Build history of the part. All positions in model axes, mm. Give positions to 0.01 mm unless a question says otherwise; leave off trailing zeros. Loops run counter-clockwise (first coordinate to the right, second up) from the corner with the lowest first, then second, coordinate; pieces in that order, holes last. Notation, with made-up numbers: M 87,17.5 L 118,17.5 A10 ccw 118,22.5 Z; hole C 66,-40 d9. An arc over 180 degrees is marked long. Put each result on its own line as item: value.
```python
from build123d import *

# Parameters (mm, degrees)
SKETCH1_R           = 4
SKETCH1_R_2         = 12
BOSS_EXTRUDE1_DEPTH = 2.5
FILLET1_R           = 4


with BuildPart() as part:
    # Sketch1 → Boss-Extrude1 (new, symmetric)
    with BuildSketch(Plane(origin=(0, 0, 0), x_dir=(1, 0, 0), z_dir=(0, 1, 0))):
        with BuildLine():
            Line((39.081081081, 10.801347209), (3.405405405, 17.674931797))
            ThreePointArc((3.405405405, 17.674931797), (0, 18), (-3.405405405, 17.674931797))
            Line((-3.405405405, 17.674931797), (-39.081081081, 10.801347209))
            ThreePointArc((-39.081081081, 10.801347209), (-48, 0), (-39.081081081, -10.801347209))
            Line((-39.081081081, -10.801347209), (-3.405405405, -17.674931797))
            ThreePointArc((-3.405405405, -17.674931797), (0, -18), (3.405405405, -17.674931797))
            Line((3.405405405, -17.674931797), (39.081081081, -10.801347209))
            ThreePointArc((39.081081081, -10.801347209), (48, 0), (39.081081081, 10.801347209))
        make_face()
        with Locations(Location((37, 0, 0), (0, 0, 270))):
            Circle(SKETCH1_R, mode=Mode.SUBTRACT)
        with Locations(Location((-37, 0, 0), (0, 0, 270))):
            Circle(SKETCH1_R, mode=Mode.SUBTRACT)
        with Locations(Location((0, 0, 0), (0, 0, 270))):
            Circle(SKETCH1_R_2, mode=Mode.SUBTRACT)
        with BuildLine():
            Line((-29.082089608, -7.635882073), (-14.68452203, -10.40984211))
            ThreePointArc((-14.68452203, -10.40984211), (-18, 0), (-14.68452203, 10.40984211))
            Line((-14.68452203, 10.40984211), (-29.082089608, 7.635882073))
            ThreePointArc((-29.082089608, 7.635882073), (-26, 0), (-29.082089608, -7.635882073))
        make_face(mode=Mode.SUBTRACT)
        with BuildLine():
            ThreePointArc((29.082089608, -7.635882073), (26, 0), (29.082089608, 7.635882073))
            Line((29.082089608, 7.635882073), (14.68452203, 10.40984211))
            ThreePointArc((14.68452203, 10.40984211), (18, 0), (14.68452203, -10.40984211))
            Line((14.68452203, -10.40984211), (29.082089608, -7.635882073))
        make_face(mode=Mode.SUBTRACT)
    extrude(amount=BOSS_EXTRUDE1_DEPTH, both=True)

    # Fillet1
    fillet1_edges = [part.edges().sort_by_distance(p)[0] for p in [
        (29.082089608, 0, -7.635882073),
        (14.68452203, 0, -10.40984211),
        (14.68452203, 0, 10.40984211),
        (29.082089608, 0, 7.635882073),
        (-14.68452203, 0, 10.40984211),
        (-14.68452203, 0, -10.40984211),
        (-29.082089608, 0, -7.635882073),
        (-29.082089608, 0, 7.635882073),
    ]]
    fillet(fillet1_edges, radius=FILLET1_R)


solid = part.part
```
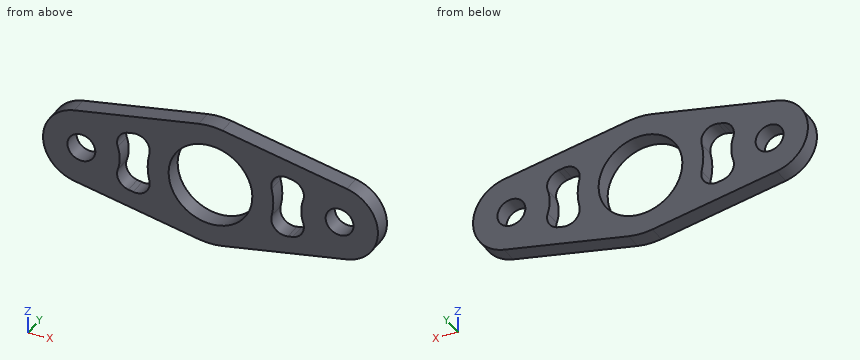
Q1. Slice it at D-D (x = 0). List the corners of the cut face in (y, z).
Here are the results:
outline: M -2.5,-18 L 2.5,-18 L 2.5,-12 L -2.5,-12 Z; M -2.5,12 L 2.5,12 L 2.5,18 L -2.5,18 Z
Q2. Slice it at A-A (z = 0). List the corners of the cut face in (x, y), and give its area (3 significant figures).
Here are the results:
outline: M -48,-2.5 L -41,-2.5 L -41,2.5 L -48,2.5 Z; M -33,-2.5 L -26,-2.5 L -26,2.5 L -33,2.5 Z; M -18,-2.5 L -12,-2.5 L -12,2.5 L -18,2.5 Z; M 12,-2.5 L 18,-2.5 L 18,2.5 L 12,2.5 Z; M 26,-2.5 L 33,-2.5 L 33,2.5 L 26,2.5 Z; M 41,-2.5 L 48,-2.5 L 48,2.5 L 41,2.5 Z
area: 200 mm²
Q3. Slice it at C-C (y = 0.95). List the corners of the cut face in (x, z), and give its area (3 significant figures).
Here are the results:
outline: M -39.08,-10.8 L -3.41,-17.67 A18 ccw 3.41,-17.67 L 39.08,-10.8 A11 ccw 39.08,10.8 L 3.41,17.67 A18 ccw -3.41,17.67 L -39.08,10.8 A11 ccw Z; hole C -37,0 d8; hole M -26.57,-3.5 A4 ccw -23.54,-8.7 L -22.17,-8.97 A4 ccw -17.52,-4.12 A18 cw -17.52,4.12 A4 ccw -22.17,8.97 L -23.54,8.7 A4 ccw -26.57,3.5 A11 cw Z; hole C 0,0 d24; hole M 17.52,-4.12 A4 ccw 22.17,-8.97 L 23.54,-8.7 A4 ccw 26.57,-3.5 A11 cw 26.57,3.5 A4 ccw 23.54,8.7 L 22.17,8.97 A4 ccw 17.52,4.12 A18 cw Z; hole C 37,0 d8
area: 1,720 mm²
Q4. Slice it at B-B (x = -37). List the corners of the cut face in (y, z).
Here are the results:
outline: M -2.5,-11.2 L 2.5,-11.2 L 2.5,-4 L -2.5,-4 Z; M -2.5,4 L 2.5,4 L 2.5,11.2 L -2.5,11.2 Z
Q5. Drop a flat-ended pin along its axis: pin 1 Ø3 at (x, z) = (4.5, -9) entering from -Y. Give the stop position or say it passes through.
Here are the results:
pin 1: through
Q6. Probe line 1 (X direction, y = -2.2, z = -2.5); line 2 (X direction, y = 0.95, z = 5); line 3 (Z direction, x = 19, y = -1.2). List the from-to ranges inside material, lowest first. Write a range as from..to.
Here are the results:
line 1: -47.71..-40.12, -33.88..-26.29, -17.83..-11.74, 11.74..17.83, 26.29..33.88, 40.12..47.71
line 2: -46.8..-26.77, -17.42..-10.91, 10.91..17.42, 26.77..46.8
line 3: -14.67..-8.23, 8.23..14.67
